```python
from build123d import *

# Parameters (mm, degrees)
EXTRUDE_1_DEPTH     = 20
SKETCH_2_R          = 1.5
CUT_EXTRUDE_1_DEPTH = 29.142494559


with BuildPart() as part:
    # 草图1 → 凸台-拉伸1 (new body)
    with BuildSketch(Plane.XY):
        Polygon((0, 0), (0, 14), (-1, 14), (-1, -1), (14, -1), (14, 0), align=None)
    extrude(amount=EXTRUDE_1_DEPTH)

    # 草图2 → 切除-拉伸1 (cut, through all)
    with BuildSketch(Plane(origin=(0, 0, 0), x_dir=(1, 0, 0), z_dir=(0, 1, 0))):
        with Locations(Location((8, -5.5, 0), (0, 0, 180))):
            Circle(SKETCH_2_R)
        with Locations((8, -14.5)):
            Circle(SKETCH_2_R)
    cut_extrude_1 = extrude(amount=-CUT_EXTRUDE_1_DEPTH, mode=Mode.SUBTRACT)

    # 镜向1: 切除-拉伸1 across plane
    add(cut_extrude_1.mirror(Plane(origin=(0, 0, 0), x_dir=(0, 0, 1), z_dir=(-0.7071067811865476, 0.7071067811865475, 0))), mode=Mode.SUBTRACT)


solid = part.part
```
The listing builds one solid part. Answer for the finished solid, in the listing's coordinates (mm). A direction names the side the tool comes from. Coordinates: 2 decimals unless noted, no trailing zeros. Order: outer loops, then holes, each group sorted by start corner. A loop starts at its lowest first (then second) coordinate and runs counter-clockwise, first axis right, second up. Notation, with made-up numbers: M 74.5,37.5 L 81.5,37.5 A27 ccw 81.5,61.5 Z; hole C 59.5,21.25 d7. An arc over 180 degrees is marked long. Answer as a JSON object with one key per item and string values. Group by question number.
1. Section A-A on y = 8 is taken. Write down the section's boundary in (x, z), then the cut area to 3 significant figures.
2. Straight lines are drawn through the part: line 1 (Z direction, x = -0.2, y = 8); line 2 (Y direction, x = -0.55, z = 5.5); line 3 (Y direction, x = 1.5, z = 7.5). For each, find the intervals that lie inside material, in ascending order.
3. Section D-D on z = 2.25 is taken. Write down the section's boundary in (x, y), then the cut area to 3 significant figures.
4. Determine the mould class of faces 1 (the flat face through (-0.2, 3.2, 20)), 2 (the flat face through (0, 7, 10)), 3 (the cylindrical face through (9.5, -0.49, 5.57)) for opening direction X: released by +X, released by -X, zero draft, split by the parting line, or undercut.
5. Flat-ended cylindrical pins translate along their axes: P1, Ø5, axis at y = 10.5, z = 9.5, coming from the +X side; P2, Ø2.5, axis at x = 8, z = 5.5, coming from the +Y side; P3, Ø7, axis at x = 7.5, z = 10, coming from the +Y side. Find the tip coordinate at first contact, or state that the pin passes through.
6. Section C-C on x = 12 is taken. Write down the section's boundary in (y, z), then the cut area to 3 significant figures.
7. Section B-B on z = 14.5 is taken. Write down the section's boundary in (x, y).
8. A tool of negligible diameter and unlimited length cuts with its end or side. For faces 4 (the flat face through (7, 0, 10)), 5 (the flat face through (-0.5, 14, 9.9)), from which of +Z, -Z, +X, -X, +Y, -Y can it reach the whole face along a straight path? Write none if from no direction.
Values follow:
{
 "1": {"outline": "M -1,0 L 0,0 L 0,4 L -1,4 Z; M -1,7 L 0,7 L 0,13 L -1,13 Z; M -1,16 L 0,16 L 0,20 L -1,20 Z", "area": "14.0 mm2"},
 "2": {"line 1": "0 to 4, 7 to 13, 16 to 20", "line 2": "-1 to 6.5, 9.5 to 14", "line 3": "-1 to 0"},
 "3": {"outline": "M -1,-1 L 14,-1 L 14,0 L 0,0 L 0,14 L -1,14 Z", "area": "29.0 mm2"},
 "4": {"face 1": "zero draft", "face 2": "released by +X", "face 3": "undercut"},
 "5": {"P1": "x = 0", "P2": "through", "P3": "y = 0"},
 "6": {"outline": "M -1,0 L 0,0 L 0,20 L -1,20 Z", "area": "20.0 mm2"},
 "7": {"outline": "M -1,-1 L 6.5,-1 L 6.5,0 L 0,0 L 0,6.5 L -1,6.5 Z; M -1,9.5 L 0,9.5 L 0,14 L -1,14 Z; M 9.5,-1 L 14,-1 L 14,0 L 9.5,0 Z"},
 "8": {"face 4": "+Z, -Z, +X, +Y", "face 5": "+Z, -Z, +X, -X, +Y"}
}
